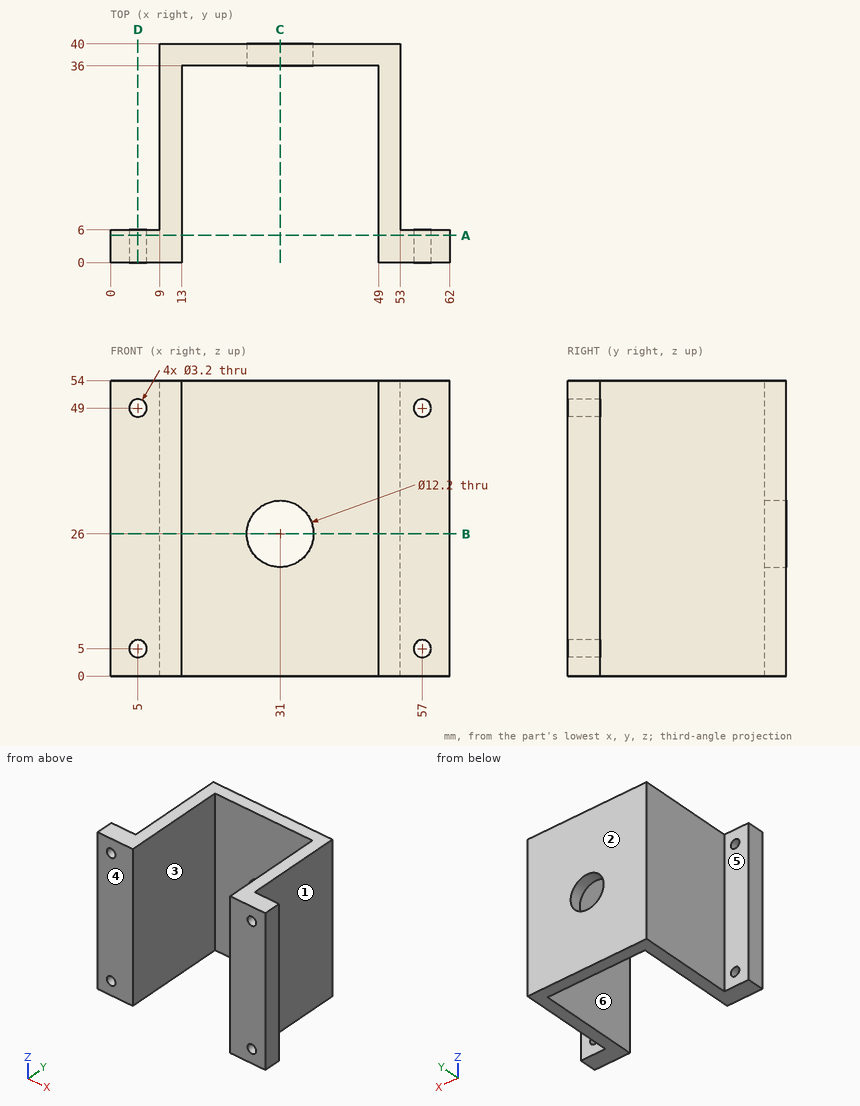
Job drawing, mm, ordinate dimensions from the low corner. One solid piece. A direction names the side the tool comes from. Coordinates: 2 decimals unless noted, no trailing zeros. Order: outer loops, then holes, each group sorted by start corner. A loop starts at its lowest first (then second) coordinate and runs counter-clockwise, first axis right, second up. Notation, with made-up numbers: (-33, 35.5) -> (-24, 35.5) arc R27 ccw to (-24, 71.5) -> close; hole circle Ø2 at (-25.75, 77). An arc over 180 degrees is marked (long way). Return JSON: item names as keys, results as strings. Group by question number.
Item 1: Flat gauge pins, fed straight in: P1, Ø8, axis at y = 23, z = 31, coming from the -X side; P2, Ø5, axis at x = 5, z = 5, coming from the +Y side; P3, Ø11, axis at x = 31, z = 26, coming from the -Y side; P4, Ø10, axis at y = 26, z = 21.5, coming from the +X side. Where does each tip first touch, or does it go through?
Item 2: Tool access for the marked faces 4, 5 and 6: list every direction of +Z, -Z, +X, -X, +Y, -Y with a clear straight run to the whole face (end or side of a thin tool).
Item 3: Pull direction X, two halves, no side cores. Call the marked faces 1, 2 and 3: pulls with the +X half, pulls with the -X half, needs draft (parallel to the pull), parting line crosses it, or undercut.
Item 4: Saw through at A-A on y = 5. Write the cut outline in (x, z), then the cut area to 3 significant figures.
Item 5: Wall check: line 1 along Z through (x, y) = (57, 1.9); line 2 along X through (y, z) = (2, 29); line 3 along X through (y, z) = (18, 17.5). Give the ranges that are in metal, low to high. Write a range as [from, to].
Item 6: Saw through at C-C on x = 31. Write the cut outline in (y, z).
Item 7: Saw through at D-D on x = 5. Write the cut outline in (y, z), then the cut area to 3 significant figures.
Item 8: Saw through at B-B on z = 26. Write the cut outline in (x, y).
Values found:
{
 "1": {"P1": "stops at x = 9", "P2": "stops at y = 6", "P3": "passes through", "P4": "stops at x = 53"},
 "2": {"face 4": "+Z, -Z, +X, -X, -Y", "face 5": "+Z, -Z, -X, +Y", "face 6": "+Z, -Z, -Y"},
 "3": {"face 1": "pulls with the +X half", "face 2": "needs draft", "face 3": "undercut"},
 "4": {"outline": "(0, 0) -> (13, 0) -> (13, 54) -> (0, 54) -> close; (49, 0) -> (62, 0) -> (62, 54) -> (49, 54) -> close; hole circle Ø3.2 at (5, 5); hole circle Ø3.2 at (5, 49); hole circle Ø3.2 at (57, 5); hole circle Ø3.2 at (57, 49)", "area": "1,370 mm2"},
 "5": {"line 1": "z = [0, 3.4], [6.6, 47.4], [50.6, 54]", "line 2": "x = [0, 13], [49, 62]", "line 3": "x = [9, 13], [49, 53]"},
 "6": {"outline": "(36, 0) -> (40, 0) -> (40, 19.9) -> (36, 19.9) -> close; (36, 32.1) -> (40, 32.1) -> (40, 54) -> (36, 54) -> close"},
 "7": {"outline": "(0, 0) -> (6, 0) -> (6, 3.4) -> (0, 3.4) -> close; (0, 6.6) -> (6, 6.6) -> (6, 47.4) -> (0, 47.4) -> close; (0, 50.6) -> (6, 50.6) -> (6, 54) -> (0, 54) -> close", "area": "286 mm2"},
 "8": {"outline": "(0, 0) -> (13, 0) -> (13, 36) -> (24.9, 36) -> (24.9, 40) -> (9, 40) -> (9, 6) -> (0, 6) -> close; (37.1, 36) -> (49, 36) -> (49, 0) -> (62, 0) -> (62, 6) -> (53, 6) -> (53, 40) -> (37.1, 40) -> close"}
}
